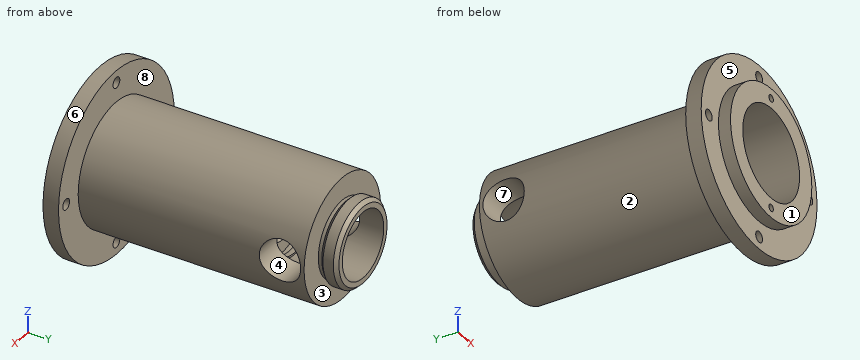
Autodesk Inventor part; units mm, degrees
ref_plane "Work Plane1" through (18.5, 0, 0) normal (1, 0, 0) x (0, 1, 0)
ref_plane "XZ Plane" through (0, 0, 0) normal (0, 1, 0) x (-1, 0, 0)
ref_plane "XY Plane" through (0, 0, 0) normal (0, 0, 1) x (1, 0, 0)
sketch "Sketch1" plane through (0, 0, 0) normal (0, 0, 1) x (1, 0, 0)
  line L0 (0, 0) -> (0, 82.5)
  line L1 (11, 82.5) -> (12, 81.5)
  line L2 (12, 81.5) -> (12, 78.5)
  line L3 (12, 78.5) -> (11, 77.5)
  line L4 (11, 77.5) -> (11, 76.5)
  line L5 (11, 76.5) -> (17.5, 76.5)
  line L6 (17.5, 76.5) -> (17.5, 11)
  line L7 (17.5, 11) -> (26.5, 11)
  line L8 (26.5, 11) -> (26.5, 6.5)
  line L9 (15, 0) -> (13, 0)
  line L10 (13, 0) -> (13, 56)
  line L11 (13, 56) -> (4, 56)
  line L12 (9.5, 62.5) -> (9.5, 82.5)
  line L13 (9.5, 82.5) -> (11, 82.5)
  line L14 (9.5, 62.5) -> (9, 62.5)
  line L15 (9, 62.5) -> (9, 61)
  line L16 (10, 59) -> (6.4, 59)
  line L17 (-4, 47) -> (4, 47)
  line L18 (4, 47) -> (4, 45)
  line L19 (4, 45) -> (-4, 45)
  line L20 (-4, 45) -> (-4, 47)
  line L21 (-4, 47) -> (4, 45) construction
  line L22 (4, 47) -> (-4, 45) construction
  line L23 (9, 61) -> (10, 61)
  line L24 (10, 61) -> (10, 59)
  line L25 (4, 56) -> (4, 56.6)
  line L26 (4, 56.6) -> (6.4, 59)
  circle A0 centre (5, 59) radius 1
  line L27 (26.5, 6.5) -> (13, 6.5)
  point P0 (0, 46)
  dimension "d0" = 26
  dimension "d1" = 35
  dimension "d8" = 56
  dimension "d11" = 24
  dimension "d14" = 135
  dimension "d15" = 22
  dimension "d16" = 22
  dimension "d18" = 3
  dimension "d22" = 19
  dimension "d26" = 135
  dimension "d28" = 6
  dimension "d30" = 18
  dimension "d38" = 8
  dimension "d39" = 2
  dimension "d50" = 14
  dimension "d59" = 20
  dimension "d60" = 2
  dimension "d61" = 3.5
  dimension "d62" = 0.6
  dimension "d63" = 3
  dimension "d64" = 2
  dimension "d65" = 10
  dimension "d66" = 8
  dimension "d67" = 135
  dimension "d68" = 53
  dimension "d69" = 11
  dimension "d70" = 4.5
revolve "Revolution1" add sketch "Sketch1" angle 360 about axis through (0, 0, 0) along (0, 1, 0) picked at (5.7132, 58.309) contours L1 L2 L3 L4 L5 L6 L7 L8 L27 L10 L11 L25 L26 A0 L16 L24 L23 L15 L14 L12 L13 | A0 L26
ref_plane "Work Plane1" through (18.5, 0, 0) normal (1, 0, 0) x (0, 1, 0)
sketch "Sketch2" plane through (18.5, 0, 0) normal (1, 0, 0) x (0, 1, 0)
  line L0 (76.5, 17.5) -> (76.5, -17.5)
  point P0 (0, 0)
  point P1 (69.5, 0)
  point P2 (76.5, 0)
  dimension "d41" = 7
hole "Hole1" at (18.5, 69.5, 0) direction (-1, 0, 0) diameter 12 end through all
thread "Thread1"
thread "Thread2"
sketch "Sketch3" plane through (0, 6.5, 0) normal (0, -1, 0) x (1, 0, 0)
  point P0 (0, 0)
  point P1 (23, 0)
  dimension "d71" = 23
hole "Hole2" at (23, 6.5, 0) direction (0, 1, 0) diameter 3.1 end through all
pattern_circular "Circular Pattern1" count 4 over 360 about axis through (0, 43.75, 0) along (0, -1, 0) of "Hole2"
sketch "Sketch4" plane through (0, 6.5, 0) normal (0, -1, 0) x (1, 0, 0)
  circle A0 centre (0, 0) radius 13
  circle A1 centre (0, 0) radius 18.5983
extrude "Extrusion1" add sketch "Sketch4" along normal blind 3.5
sketch "Sketch5" plane through (0, 3, 0) normal (0, -1, 0) x (1, 0, 0)
  circle A0 centre (0, 0) radius 18.5983
  circle A1 centre (0, 0) radius 13
  circle A2 centre (0, 0) radius 13
  line L0 (0, 13) -> (0, 18.5983)
  circle A3 centre (0, 0) radius 18.5983
  line L1 (0, -18.5983) -> (0, -13)
  point P0 (0, 0)
  point P1 (0, 15.7991)
  point P2 (0, -15.7991)
hole "Hole3" at (0, 3, 15.7991) at (0, 3, -15.7991) direction (0, 1, 0) diameter 2.013 depth 5 tip angle 118
equation "\"d14\" = d13"
properties part number "013" material "Stainless Steel, Austenitic"
Read the model definition and answer for the solid it produces. Units are mm, in the model's axes. Face numbers are marked on the shaded views. A direction names the side the tool comes from. Round coordinates to 2 decimals unless told otherwise and drop trailing zeros. Loops run counter-clockwise (first coordinate to the right, second up) from the corner with the lowest first, then second, coordinate; pieces in that order, holes last. Notation, with made-up numbers: (46, 51) -> (93, 51) arc R24 cw to (93, 79) -> close; hole circle Ø4 at (-18.75, -11.75). An arc over 180 degrees is marked (long way). One line per item, written item: value.
1) A cutting plane is placed at D-D (z = 0). Give the number of separate pieces and of enclosed holes in the cut face, and give its area (3 significant figures).
Answer list:
separate pieces: 6
enclosed holes: 0
area: 727 mm²
2) A cutting plane is placed at C-C (x = 14.5). Determine the outline of the cut face in (y, z).
Answer list:
outline: (3, -11.65) -> (6.5, -11.65) -> (6.5, -22.18) -> (11, -22.18) -> (11, -9.8) -> (76.5, -9.8) -> (76.5, 9.8) -> (11, 9.8) -> (11, 22.18) -> (6.5, 22.18) -> (6.5, 11.65) -> (3, 11.65) -> close; hole circle Ø12 at (69.5, 0)
3) A cutting plane is placed at A-A (y = 69.5). Determine the outline of the cut face in (x, z), and give its area (3 significant figures).
Answer list:
outline: (-16.44, -6) arc R17.5 ccw to (16.44, -6) -> (7.37, -6) arc R9.5 cw to (-7.37, -6) -> close; (-16.44, 6) -> (-7.37, 6) arc R9.5 cw to (7.37, 6) -> (16.44, 6) arc R17.5 ccw to start
area: 479 mm²
4) Flat-ended cylindrical pins translate along their axes: P1, Ø10, axis at x = 1, y = 72.5, coming from the -Z side; P2, Ø5, axis at x = 12, y = 22, coming from the +Z side; P3, Ø10.5, axis at x = 0, z = 0, coming from the +Y side; P4, Ø9.5, axis at y = 69.5, z = 0, coming from the +X side. Find the tip coordinate at first contact, or state that the pin passes through.
Answer list:
P1: stops at z = -17.5
P2: stops at z = 14.7
P3: stops at y = 57.85
P4: passes through
5) A cutting plane is placed at B-B (z = 23). Determine the outline of the cut face in (x, y), and give its area (3 significant figures).
Answer list:
outline: (-13.16, 6.5) -> (-1.55, 6.5) -> (-1.55, 11) -> (-13.16, 11) -> close; (1.55, 6.5) -> (13.16, 6.5) -> (13.16, 11) -> (1.55, 11) -> close
area: 105 mm²
6) For the marked faces 1, 2, 3, 4 and 5, determine the directions among +Z, -Z, +X, -X, +Y, -Y from which every point of the face is accessible in a straight line to the end or side of a thin tool.
Answer list:
face 1: +Z, -Z, +X, -X, -Y
face 2: +Y
face 3: none
face 4: +X, -X
face 5: -Y
7) The mould has two halves that part along Y. Classify the marked faces 6, 7 and 8: pulls with the +Y half, pulls with the -Y half, needs draft (parallel to the pull), parting line crosses it, or undercut.
Answer list:
face 6: needs draft
face 7: undercut
face 8: pulls with the +Y half
8) Consider L1, parallel to X at y = 8.65, z = 0; L2, parallel to Y at x = 12.5, z = 0; L3, parallel to X at y = 77, z = 0. Determine where each line is inside the solid, lowest interval first. Write a range as [from, to].
Answer list:
L1: x = [-26.5, -24.55], [-21.45, -13], [13, 21.45], [24.55, 26.5]
L2: y = [56, 63.5], [75.5, 76.5]
L3: x = [-11, -9.5], [9.5, 11]
